```python
from build123d import *

# Parameters (mm, degrees)
SKETCH_1_R          = 1.5
EXTRUDE_1_DEPTH     = 45
CUT_EXTRUDE_1_DEPTH = 10
SKETCH_3_R          = 3
EXTRUDE_2_DEPTH     = 5
SKETCH_4_R          = 40
EXTRUDE_3_DEPTH     = 35


with BuildPart() as part:
    # 草图1 → 凸台-拉伸1 (new body)
    with BuildSketch(Plane(origin=(0, 0, 0), x_dir=(1, 0, 0), z_dir=(0, 1, 0))):
        Polygon((42.5, 35), (42.5, 15), (47.5, 5), (47.5, -35), (-47.5, -35), (-47.5, 35), align=None)
        with Locations((-39.5, -27)):
            Circle(SKETCH_1_R, mode=Mode.SUBTRACT)
        with Locations((-23.5, -27)):
            Circle(SKETCH_1_R, mode=Mode.SUBTRACT)
        with Locations((-7.5, -27)):
            Circle(SKETCH_1_R, mode=Mode.SUBTRACT)
        with Locations((8.5, -27)):
            Circle(SKETCH_1_R, mode=Mode.SUBTRACT)
        with Locations((24.5, -27)):
            Circle(SKETCH_1_R, mode=Mode.SUBTRACT)
        with Locations((-23.5, 5)):
            Circle(SKETCH_1_R, mode=Mode.SUBTRACT)
        with Locations((-7.5, 5)):
            Circle(SKETCH_1_R, mode=Mode.SUBTRACT)
        with Locations((8.5, 5)):
            Circle(SKETCH_1_R, mode=Mode.SUBTRACT)
        with Locations((24.5, 5)):
            Circle(SKETCH_1_R, mode=Mode.SUBTRACT)
        with Locations((-39.5, 5)):
            Circle(SKETCH_1_R, mode=Mode.SUBTRACT)
    extrude(amount=EXTRUDE_1_DEPTH)

    # 草图2 → 切除-拉伸1 (cut)
    with BuildSketch(Plane(origin=(42.5, 0, 0), x_dir=(0, 0, -1), z_dir=(1, 0, 0))):
        Polygon((15, 29.001286667), (23.488716393, 29.001286667), (23.488716393, 24.069127899), (25.866721513, 24.069127899), (25.866721513, 18.87274634), (23.488716393, 18.87274634), (23.488716393, 14.028661836), (15, 14.028661836), align=None)
    extrude(amount=-CUT_EXTRUDE_1_DEPTH, mode=Mode.SUBTRACT)

    # 草图3 → 凸台-拉伸2 (add)
    with BuildSketch(Plane.ZY.offset(47.5)):
        with Locations((19, 22.5)):
            Circle(SKETCH_3_R)
    extrude(amount=EXTRUDE_2_DEPTH)

    # 草图4 → 凸台-拉伸3 (add)
    with BuildSketch(Plane.ZY.offset(52.5)):
        with Locations((19, 22.5)):
            Circle(SKETCH_4_R)
    extrude(amount=EXTRUDE_3_DEPTH)


solid = part.part
```
Could you check a few things on this model? Use its own coordinates, in mm. A direction names the side the tool comes from. Round coordinates to 2 decimals unless told otherwise and drop trailing zeros. Write each loop counter-clockwise with the first axis right and the second up, starting at its lowest first coordinate (ties: lowest second). Pieces come first, ordered by that corner, then holes. Notation, with made-up numbers: M -11.75,50.25 L 1.25,50.25 A14 cw 1.25,54.25 Z; hole C -29,86 d10. An arc over 180 degrees is marked long. Answer in a Markdown table with one row per item. Add a question column.
Q1. Imagine slicing it at C-C (x = -39.5). Please give me the cut outline in (y, z).
Q2. Imagine slicing it at A-A (y = 31.5). Give the number of separate pieces and of enclosed holes in the cut face, then the cut area to 3 significant figures.
Q3. On a 3-axis mill with a long thin cutter (end or side, diameter ignored), from which of +Z, -Z, +X, -X, +Y, -Y can I reach the whole of each face in a straight line? I mean faces 4 (the flat face through (1, 45, 0)), 5 (the cylindrical face through (-50, 22.6, 16)), 6 (the flat face through (38, 21, -15)), 7 (the flat face through (42.5, 22, -27)). Say none if no direction works.
Q4. Imagine slicing it at D-D (x = 35.5). Please give me the cut outline in (y, z), then the cut area to 3 significant figures.
Q5. Will these pins go through, and if not, where does the flat tip stop? pin 1 Ø5 at (x, z) = (-60.5, 14.5) entering from -Y; pin 2 Ø4 at (x, z) = (36, -20) entering from +Y; pin 3 Ø3.5 at (x, z) = (24.5, 27) entering from -Y.
Q6. If we mould it in two halves opening along Z, with no side actions, what happens to faces 1 (the flat face through (1, 0, 0)), 2 (the flat face through (45, 22, -10)), 3 (the cylindrical face through (-25, 22, -5))? For each: +Z half, -Z half, draft (parallel to the pull), parting line (faces both ways), or undercut.
Q7. If I drill on line 1 (Z direction, x = 24.5, y = 34); line 2 (X direction, y = 0.5, z = 2); line 3 (Z direction, x = -39, y = 22), over which ranges is the centre line in solid material (lowest first)? Write a range as from..to.
Q8. Imagine slicing it at B-B (z = -19). Please give me the cut outline in (x, y), then the cut area to 3 significant figures.
Values:
| question | item | result |
|---|---|---|
| 1 | outline | M 0,-35 L 45,-35 L 45,-6.5 L 0,-6.5 Z; M 0,-3.5 L 45,-3.5 L 45,25.5 L 0,25.5 Z; M 0,28.5 L 45,28.5 L 45,35 L 0,35 Z |
| 2 | separate pieces | 2 |
| 2 | enclosed holes | 10 |
| 2 | area | 9,180 mm^2 |
| 3 | face 4 | +Z, -Z, +X, +Y |
| 3 | face 5 | none |
| 3 | face 6 | +X |
| 3 | face 7 | -Z, +X, +Y, -Y |
| 4 | outline | M 0,-35 L 45,-35 L 45,35 L 0,35 Z; hole M 14.03,-23.49 L 18.87,-23.49 L 18.87,-25.87 L 24.07,-25.87 L 24.07,-23.49 L 29,-23.49 L 29,-15 L 14.03,-15 Z |
| 4 | area | 3,010 mm^2 |
| 5 | pin 1 | y = -17.45 |
| 5 | pin 2 | y = 45 |
| 5 | pin 3 | y = 0 |
| 6 | face 1 | draft |
| 6 | face 2 | -Z half |
| 6 | face 3 | undercut |
| 7 | line 1 | -35..-6.5, -3.5..25.5, 28.5..35 |
| 7 | line 2 | -87.5..-52.5, -47.5..47.5 |
| 7 | line 3 | -35..-6.41, -3.59..25.59, 28.41..35 |
| 8 | outline | M -87.5,10.01 L -52.5,10.01 L -52.5,34.99 L -87.5,34.99 Z; M -47.5,0 L 42.5,0 L 42.5,14.03 L 32.5,14.03 L 32.5,29 L 42.5,29 L 42.5,45 L -47.5,45 Z |
| 8 | area | 4,770 mm^2 |
